```python
from build123d import *

# Parameters (mm, degrees)
SKETCH1_W                = 200
SKETCH1_H                = 200
SKETCH1_R                = 0.0005
BOSS_EXTRUDE1_DEPTH      = 10
SKETCH2_W                = 30
SKETCH2_H                = 5
CUT_EXTRUDE1_DEPTH       = 5
BOSS_EXTRUDE3_START      = 15
BOSS_EXTRUDE3_DEPTH      = 5
CIRPATTERN1_COUNT        = 4
CIRPATTERN1_START        = 15
CIRPATTERN1_COPY_1_DEPTH = 5
CIRPATTERN1_COPY_2_DEPTH = 5
CIRPATTERN1_COPY_3_DEPTH = 5
SKETCH4_W                = 160
SKETCH4_H                = 160
CUT_EXTRUDE2_DEPTH       = 10


with BuildPart() as part:
    # Sketch1 → Boss-Extrude1 (new body)
    with BuildSketch(Plane(origin=(0, 0, 0), x_dir=(1, 0, 0), z_dir=(0, 1, 0))):
        Rectangle(SKETCH1_W, SKETCH1_H)
        with Locations(Location((0, 0, 0), (0, 0, 270))):
            Circle(SKETCH1_R, mode=Mode.SUBTRACT)
    extrude(amount=BOSS_EXTRUDE1_DEPTH)

    # Sketch2 → Cut-Extrude1 (cut)
    with BuildSketch(Plane(origin=(0, 10, 0), x_dir=(1, 0, 0), z_dir=(0, 1, 0))):
        with Locations((45, 97.5)):
            Rectangle(SKETCH2_W, SKETCH2_H)
        with Locations((-45, 97.5)):
            Rectangle(SKETCH2_W, SKETCH2_H)
    cut_extrude1 = extrude(amount=-CUT_EXTRUDE1_DEPTH, mode=Mode.SUBTRACT)

    # Sketch3 → Boss-Extrude3 (add)
    with BuildSketch(Plane.ZY.offset(-60).offset(BOSS_EXTRUDE3_START)):
        with BuildLine():
            Line((-97.5, 10), (-95, 10))
            ThreePointArc((-95, 10), (-103.535533906, 13.535533906), (-100, 5))
            Line((-100, 5), (-100, 7.5))
            ThreePointArc((-100, 7.5), (-101.767766953, 11.767766953), (-97.5, 10))
        make_face()
        with BuildLine():
            ThreePointArc((-100, 5), (-96.464466094, 6.464466094), (-95, 10))
            Line((-95, 10), (-97.5, 10))
            ThreePointArc((-97.5, 10), (-98.232233047, 8.232233047), (-100, 7.5))
            Line((-100, 7.5), (-100, 5))
        make_face()
        with BuildLine():
            Line((-95, 5), (-95, 10))
            ThreePointArc((-95, 10), (-96.464466094, 6.464466094), (-100, 5))
            Line((-100, 5), (-95, 5))
        make_face()
    boss_extrude3 = extrude(amount=BOSS_EXTRUDE3_DEPTH)

    # Mirror1: Boss-Extrude3 across plane
    add(boss_extrude3.mirror(Plane(origin=(0, 0, 0), x_dir=(0, 0, 1), z_dir=(1, 0, 0))))

    # CirPattern1: Cut-Extrude1, Boss-Extrude3 ×4 about axis
    cirpattern1_axis = Axis((0, 0, 0), (0, 1, 0))
    add([cut_extrude1.rotate(cirpattern1_axis, i * 360 / CIRPATTERN1_COUNT) for i in range(1, CIRPATTERN1_COUNT)], mode=Mode.SUBTRACT)
    add([boss_extrude3.rotate(cirpattern1_axis, i * 360 / CIRPATTERN1_COUNT) for i in range(1, CIRPATTERN1_COUNT)])

    # CirPattern1 copy 1 sketch → CirPattern1 copy 1 (add)
    with BuildSketch(Plane(origin=(0, 0, 60), x_dir=(1, 0, 0), z_dir=(0, 0, -1)).offset(CIRPATTERN1_START)):
        with BuildLine():
            Line((-97.5, -10), (-95, -10))
            ThreePointArc((-95, -10), (-103.535533906, -13.535533906), (-100, -5))
            Line((-100, -5), (-100, -7.5))
            ThreePointArc((-100, -7.5), (-101.767766953, -11.767766953), (-97.5, -10))
        make_face()
        with BuildLine():
            ThreePointArc((-100, -5), (-96.464466094, -6.464466094), (-95, -10))
            Line((-95, -10), (-97.5, -10))
            ThreePointArc((-97.5, -10), (-98.232233047, -8.232233047), (-100, -7.5))
            Line((-100, -7.5), (-100, -5))
        make_face()
        with BuildLine():
            Line((-95, -5), (-95, -10))
            ThreePointArc((-95, -10), (-96.464466094, -6.464466094), (-100, -5))
            Line((-100, -5), (-95, -5))
        make_face()
    extrude(amount=CIRPATTERN1_COPY_1_DEPTH)

    # CirPattern1 copy 2 sketch → CirPattern1 copy 2 (add)
    with BuildSketch(Plane(origin=(60, 0, 0), x_dir=(0, 0, -1), z_dir=(-1, 0, 0)).offset(CIRPATTERN1_START)):
        with BuildLine():
            Line((-97.5, -10), (-95, -10))
            ThreePointArc((-95, -10), (-103.535533906, -13.535533906), (-100, -5))
            Line((-100, -5), (-100, -7.5))
            ThreePointArc((-100, -7.5), (-101.767766953, -11.767766953), (-97.5, -10))
        make_face()
        with BuildLine():
            ThreePointArc((-100, -5), (-96.464466094, -6.464466094), (-95, -10))
            Line((-95, -10), (-97.5, -10))
            ThreePointArc((-97.5, -10), (-98.232233047, -8.232233047), (-100, -7.5))
            Line((-100, -7.5), (-100, -5))
        make_face()
        with BuildLine():
            Line((-95, -5), (-95, -10))
            ThreePointArc((-95, -10), (-96.464466094, -6.464466094), (-100, -5))
            Line((-100, -5), (-95, -5))
        make_face()
    extrude(amount=CIRPATTERN1_COPY_2_DEPTH)

    # CirPattern1 copy 3 sketch → CirPattern1 copy 3 (add)
    with BuildSketch(Plane(origin=(0, 0, -60), x_dir=(-1, 0, 0), z_dir=(0, 0, 1)).offset(CIRPATTERN1_START)):
        with BuildLine():
            Line((-97.5, -10), (-95, -10))
            ThreePointArc((-95, -10), (-103.535533906, -13.535533906), (-100, -5))
            Line((-100, -5), (-100, -7.5))
            ThreePointArc((-100, -7.5), (-101.767766953, -11.767766953), (-97.5, -10))
        make_face()
        with BuildLine():
            ThreePointArc((-100, -5), (-96.464466094, -6.464466094), (-95, -10))
            Line((-95, -10), (-97.5, -10))
            ThreePointArc((-97.5, -10), (-98.232233047, -8.232233047), (-100, -7.5))
            Line((-100, -7.5), (-100, -5))
        make_face()
        with BuildLine():
            Line((-95, -5), (-95, -10))
            ThreePointArc((-95, -10), (-96.464466094, -6.464466094), (-100, -5))
            Line((-100, -5), (-95, -5))
        make_face()
    extrude(amount=CIRPATTERN1_COPY_3_DEPTH)

    # Sketch4 → Cut-Extrude2 (cut)
    with BuildSketch(Plane(origin=(0, 10, 0), x_dir=(1, 0, 0), z_dir=(0, 1, 0))):
        Rectangle(SKETCH4_W, SKETCH4_H)
    extrude(amount=-CUT_EXTRUDE2_DEPTH, mode=Mode.SUBTRACT)


solid = part.part
```
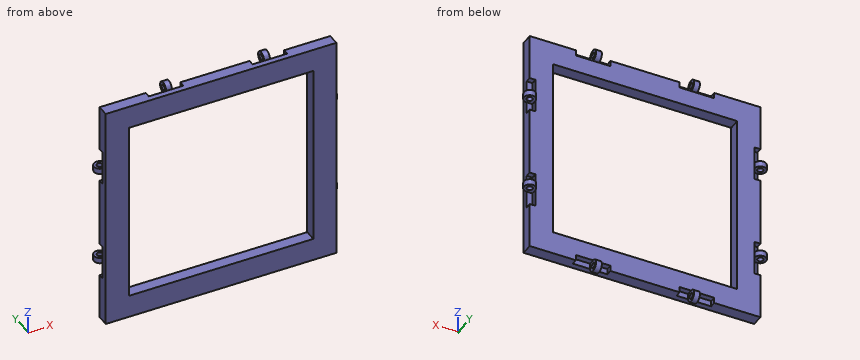
Work out the finished part from the listing and answer in its coordinate system (mm). Round coordinates to 2 decimals unless told otherwise and drop trailing zeros. Write each loop counter-clockwise with the first axis right and the second up, starting at its lowest first coordinate (ties: lowest second). Pieces come first, ordered by that corner, then holes.
1) A cutting plane is placed at C-C on x = 57. Determine the outline of the cut face in (y, z).
2) A cutting plane is placed at D-D on z = -91. Determine the outline of the cut face in (x, y).
3) A cutting plane is placed at A-A on z = 74. Determine the outline of the cut face in (x, y), and give its area (3 significant figures).
4) A cutting plane is placed at B-B on x = -8. Determine the outline of the cut face in (y, z), and give its area (3 significant figures).
5) Flat-ended cylindrical pins translate along their axes: P1, Ø5.5, axis at x = -52, y = 6.5, coming from the -Z side; P2, Ø2.5, axis at y = 8, z = -35.5, coming from the +X side; P3, Ø1.5, axis at x = 33.5, z = -98, coming from the +Y side. Find the tip coordinate at first contact, or state that the pin passes through.
6) Consider probe 1 along X at (y, z) = (2.5, 43); probe 2 along X at (y, z) = (9.5, 50). Determine where each line is inside the solid, lowest interval first.
Entries:
1. outline: (0, -100) - (5, -100) - (5, -95) - (10, -95) - (10, -80) - (0, -80) - close; (0, 80) - (10, 80) - (10, 95) - (5, 95) - (5, 100) - (0, 100) - close
2. outline: (-100, 0) - (100, 0) - (100, 10) - (-100, 10) - close
3. outline: (-100, 0) - (-80, 0) - (-80, 10) - (-100, 10) - close; (80, 0) - (100, 0) - (100, 10) - (80, 10) - close
3. area: 400 mm2
4. outline: (0, -100) - (10, -100) - (10, -80) - (0, -80) - close; (0, 80) - (10, 80) - (10, 100) - (0, 100) - close
4. area: 400 mm2
5. P1: stops at z = -100
5. P2: stops at x = 95
5. P3: stops at y = 5
6. probe 1: x = -100 to -80, 80 to 100
6. probe 2: x = -95 to -80, 80 to 95
